```python
from build123d import *

# Parameters (mm, degrees)
SKETCH1_R                = 5
BOSS_EXTRUDE1_DEPTH      = 5
BOSS_EXTRUDE2_DEPTH      = 25
BOSS_EXTRUDE2_DEPTH_BACK = 5
SKETCH2_R                = 5


with BuildPart() as part:
    # Sketch1 → Boss-Extrude1 (new, symmetric)
    with BuildSketch(Plane(origin=(0, 0, 0), x_dir=(1, 0, 0), z_dir=(0, 1, 0))):
        with BuildLine():
            Line((-55, -10), (55, -10))
            ThreePointArc((55, -10), (65, 0), (55, 10))
            Line((55, 10), (-55, 10))
            ThreePointArc((-55, 10), (-65, 0), (-55, -10))
        make_face()
        with Locations(Location((-55, 0, 0), (0, 0, 270))):
            Circle(SKETCH1_R, mode=Mode.SUBTRACT)
        with Locations(Location((55, 0, 0), (0, 0, 270))):
            Circle(SKETCH1_R, mode=Mode.SUBTRACT)
    extrude(amount=BOSS_EXTRUDE1_DEPTH, both=True)

    # Sketch2 → Boss-Extrude2 (add, two sides: drawn at the far end of the back side and taken through both)
    with BuildSketch(Plane(origin=(0, 0, 0), x_dir=(1, 0, 0), z_dir=(0, 1, 0)).offset(-BOSS_EXTRUDE2_DEPTH_BACK)):
        with Locations(Location((-55, 0, 0), (0, 0, 270))):
            Circle(SKETCH2_R)
    extrude(amount=BOSS_EXTRUDE2_DEPTH + BOSS_EXTRUDE2_DEPTH_BACK)


solid = part.part
```
Read the model definition and answer for the solid it produces. Units are mm, in the model's axes. A direction names the side the tool comes from. Give positions to 0.01 mm unless a question says otherwise; leave off trailing zeros. Write each loop counter-clockwise with the first axis right and the second up, starting at its lowest first coordinate (ties: lowest second). Pieces come first, ordered by that corner, then holes. Notation, with made-up numbers: (49, 26.5) -> (103, 26.5) arc R14 ccw to (103, 31.5) -> close; hole circle Ø3 at (-15.75, 70.5). An arc over 180 degrees is marked (long way). Answer as a JSON object with one key per item and string values.
1) Straight lines are drawn through the part: probe 1 along X at (y, z) = (-1, 0); probe 2 along Y at (x, z) = (31, -6); probe 3 along X at (y, z) = (5.5, 4.5). For each, find the intervals that lie inside material, in ascending order. Write a range as from..to.
Findings below:
{"probe 1": "x = -65..50, 60..65", "probe 2": "y = -5..5", "probe 3": "x = -57.18..-52.82"}
2) A tool of negligible diameter and unlimited length cuts with its end or side. For faces 1 (the cylindrical face through (-65, 0, 0)), 2 (the cylindrical face through (-50.043, 14.86, -0.651)), from which of +Z, -Z, +X, -X, +Y, -Y can it reach the whole face along a straight path? Write none if from no direction.
Findings below:
{"face 1": "-X, +Y, -Y", "face 2": "+Y"}
3) Section B-B on y = 2 is taken. Write down the section's boundary in (x, z).
Findings below:
{"outline": "(-55, -10) -> (55, -10) arc R10 ccw to (55, 10) -> (-55, 10) arc R10 ccw to start; hole circle Ø10 at (55, 0)"}
4) For a pull along Z with two mould halves and no side action, classify faces 3 (the flat face through (-1, 0, 10)), 4 (the cylindrical face through (65, 0, 0)), 5 (the cylindrical face through (59.957, -0.07, -0.651)), 6 (the flat face through (-1, -5, 0)) as pulls with the +Z half, pulls with the -Z half, needs draft (parallel to the pull), parting line crosses it, or undercut.
Findings below:
{"face 3": "pulls with the +Z half", "face 4": "parting line crosses it", "face 5": "undercut", "face 6": "needs draft"}
5) Section A-A on z = 0 is taken. Write down the section's boundary in (x, y), then the cut area to 3 significant figures.
Findings below:
{"outline": "(-65, -5) -> (50, -5) -> (50, 5) -> (-50, 5) -> (-50, 25) -> (-60, 25) -> (-60, 5) -> (-65, 5) -> close; (60, -5) -> (65, -5) -> (65, 5) -> (60, 5) -> close", "area": "1,400 mm^2"}
6) Section C-C on x = -53 is taken. Write down the section's boundary in (y, z), then the cut area to 3 significant figures.
Findings below:
{"outline": "(-5, -10) -> (5, -10) -> (5, -4.58) -> (25, -4.58) -> (25, 4.58) -> (5, 4.58) -> (5, 10) -> (-5, 10) -> close", "area": "383 mm^2"}
7) Section D-D on y = 21 is taken. Write down the section's boundary in (x, z), then the cut area to 3 significant figures.
Findings below:
{"outline": "circle Ø10 at (-55, 0)", "area": "78.5 mm^2"}
8) Flat-ended cylindrical pins translate along their axes: pin 1 Ø10 at (x, z) = (40, -4) entering from +Y; pin 2 Ø10 at (y, z) = (12.5, 6) entering from +X; pin 3 Ø4 at (y, z) = (16, 6.5) entering from +X. Find the tip coordinate at first contact, or state that the pin passes through.
Findings below:
{"pin 1": "stops at y = 5", "pin 2": "stops at x = -50.1", "pin 3": "stops at x = -52.82"}
